from build123d import *

# Parameters (mm, degrees)
ESQUISSE1_W        = 134
ESQUISSE1_H        = 10
ESQUISSE1_R        = 2.5
ESQUISSE1_W_2      = 5
ESQUISSE1_H_2      = 4
BOSS_EXTRU_1_DEPTH = 10
ESQUISSE1_3_R      = 2.5
BOSS_EXTRU_2_DEPTH = 13
CONG_2_R           = 1
CONG_3_R           = 1
ESQUISSE1_4_W      = 20
ESQUISSE1_4_H      = 2
BOSS_EXTRU_3_DEPTH = 2
CONG_4_R           = 1


with BuildPart() as part:
    # Esquisse1 → Boss.-Extru.1 (new body)
    # profile 1 of 5: a face of its own
    with BuildSketch(Plane.XY):
        with Locations((-99.758882294, 67.500907441)):
            Rectangle(ESQUISSE1_W, ESQUISSE1_H)
        with Locations((-96.758882294, 67.500907441)):
            Circle(ESQUISSE1_R, mode=Mode.SUBTRACT)
    # profile 2 of 5: a face of its own
    with BuildSketch(Plane.XY):
        with BuildLine():
            Line((-166.758882294, 72.500907441), (-206.758882294, 68.000907441))
            ThreePointArc((-206.758882294, 68.000907441), (-234.758882294, -12.499092559), (-206.758882294, -92.999092559))
            Line((-206.758882294, -92.999092559), (-166.758882294, -97.499092559))
            Line((-166.758882294, -97.499092559), (-166.758882294, -87.499092559))
            Line((-166.758882294, -87.499092559), (-206.758882294, -82.999092559))
            ThreePointArc((-206.758882294, -82.999092559), (-224.758882294, -12.499092559), (-206.758882294, 58.000907441))
            Line((-206.758882294, 58.000907441), (-166.758882294, 62.500907441))
            Line((-166.758882294, 62.500907441), (-166.758882294, 72.500907441))
        make_face()
        with Locations((-229.758882294, -12.499092559)):
            Circle(ESQUISSE1_R, mode=Mode.SUBTRACT)
    # profile 3 of 5: a face of its own
    with BuildSketch(Plane.XY):
        with Locations((-99.758882294, -92.499092559)):
            Rectangle(ESQUISSE1_W, ESQUISSE1_H)
        with Locations((-96.758882294, -92.499092559)):
            Circle(ESQUISSE1_R, mode=Mode.SUBTRACT)
    # profile 4 of 5: a face of its own
    with BuildSketch(Plane.XY):
        with Locations((-30.258882294, 67.500907441)):
            Rectangle(ESQUISSE1_W_2, ESQUISSE1_H_2)
    # profile 5 of 5: a face of its own
    with BuildSketch(Plane.XY):
        with Locations((-30.258882294, -92.499092559)):
            Rectangle(ESQUISSE1_W_2, ESQUISSE1_H_2)
    extrude(amount=BOSS_EXTRU_1_DEPTH)

    # Esquisse1_3 → Boss.-Extru.2 (add)
    with BuildSketch(Plane.XY):
        with Locations(Location((-96.758882294, 67.500907441, 0), (0, 0, 180))):
            Circle(ESQUISSE1_3_R)
        with Locations(Location((-229.758882294, -12.499092559, 0), (0, 0, 180))):
            Circle(ESQUISSE1_3_R)
        with Locations(Location((-96.758882294, -92.499092559, 0), (0, 0, 180))):
            Circle(ESQUISSE1_3_R)
    extrude(amount=BOSS_EXTRU_2_DEPTH)

    # Cong_2
    cong_2_edges = [part.edges().sort_by_distance(p)[0] for p in [
        (-94.258882294, -92.499092559, 13),
    ]]
    fillet(cong_2_edges, radius=CONG_2_R)

    # Cong_3
    cong_3_edges = [part.edges().sort_by_distance(p)[0] for p in [
        (-94.258882294, 67.500907441, 13),
        (-227.258882294, -12.499092559, 13),
    ]]
    fillet(cong_3_edges, radius=CONG_3_R)

    # Esquisse1_4 → Boss.-Extru.3 (add)
    with BuildSketch(Plane.XY):
        with Locations((-148.758882294, -86.499092559)):
            Rectangle(ESQUISSE1_4_W, ESQUISSE1_4_H)
        with Locations((-148.758882294, 61.500907441)):
            Rectangle(ESQUISSE1_4_W, ESQUISSE1_4_H)
    extrude(amount=BOSS_EXTRU_3_DEPTH)

    # Cong_4
    cong_4_edges = [part.edges().sort_by_distance(p)[0] for p in [
        (-148.758882294, -85.499092559, 0),
        (-148.758882294, 60.500907441, 0),
    ]]
    fillet(cong_4_edges, radius=CONG_4_R)


solid = part.part
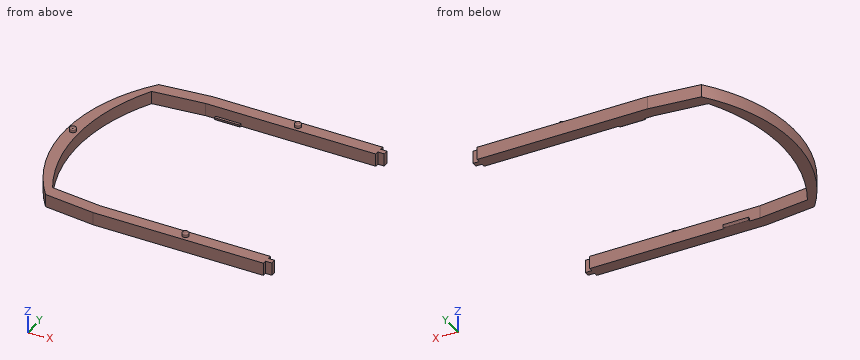
Work out the finished part from the listing and answer in its coordinate system (mm). Coordinates: 2 decimals unless noted, no trailing zeros. Loops run counter-clockwise (first coordinate to the right, second up) from the corner with the lowest first, then second, coordinate; pieces in that order, holes last. Notation, with made-up numbers: M 33,-24 L 84,-24 A21 cw 84,12 Z; hole C 8,-28 d11. An arc over 180 degrees is marked long. Answer in a Markdown table with one row per item. Add a question column.
1. Flat-ended cylindrical pins translate along their axes: P1, Ø0.6, axis at y = -87, z = 1, coming from the +X side; P2, Ø1, axis at y = 61.5, z = 1, coming from the -X side; P3, Ø5, axis at x = -173, z = 9, coming from the -Y side. Find the tip coordinate at first contact, or state that the pin passes through.
2. Find section D-D, the plane y = 7.5. Write down the section's boundary in (x, z), then the cut area to 3 significant figures.
3. Consider L1, parallel to Y at x = -74.5, z = 3.5; L2, parallel to Y at x = -209, z = 7.5; L3, parallel to X at y = 8, z = 5.25. Determine where each line is inside the solid, lowest interval first.
4. Find section A-A, the plane z = 7.75. Write down the section's boundary in (x, y) (1 decimal).
5. Find section C-C, the plane x = -190. Write down the section's boundary in (y, z), then the cut area to 3 significant figures.
6. Find section B-B, the plane x = -212.5. Write down the section's boundary in (y, z).
Reported:
| question | item | result |
|---|---|---|
| 1 | P1 | stops at x = -138.76 |
| 1 | P2 | stops at x = -211.93 |
| 1 | P3 | stops at y = -97.08 |
| 2 | outline | M -233.21,0 L -223.39,0 L -223.39,10 L -233.21,10 Z |
| 2 | area | 98.2 mm^2 |
| 3 | L1 | y = -97.5 to -87.5, 62.5 to 72.5 |
| 3 | L2 | y = -90.08 to -78.73, 53.73 to 65.09 |
| 3 | L3 | x = -233.13 to -223.32 |
| 4 | outline | M -206.8,-93 L -166.8,-97.5 L -32.8,-97.5 L -32.8,-94.5 L -27.8,-94.5 L -27.8,-90.5 L -32.8,-90.5 L -32.8,-87.5 L -166.8,-87.5 L -206.8,-83 A147.1 cw -206.8,58 L -166.8,62.5 L -32.8,62.5 L -32.8,65.5 L -27.8,65.5 L -27.8,69.5 L -32.8,69.5 L -32.8,72.5 L -166.8,72.5 L -206.8,68 A129.7 ccw Z |
| 5 | outline | M -94.88,0 L -84.88,0 L -84.88,10 L -94.88,10 Z; M 59.89,0 L 69.89,0 L 69.89,10 L 59.89,10 Z |
| 5 | area | 200 mm^2 |
| 6 | outline | M -85.16,0 L -71.28,0 L -71.28,10 L -85.16,10 Z; M 46.28,0 L 60.16,0 L 60.16,10 L 46.28,10 Z |
